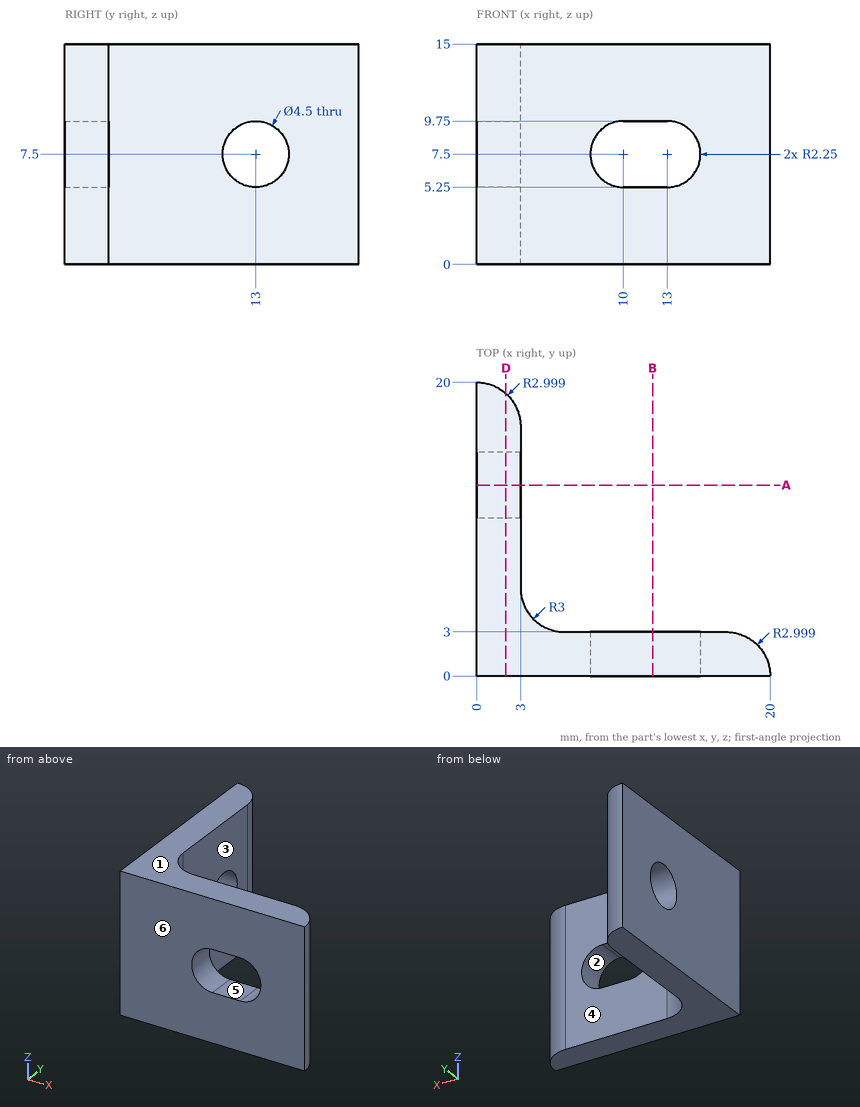
Geometry: see drawing. Coordinates: mm, zero at the bounding-box minimum. A direction names the side the tool comes from. Coordinates: 2 decimals unless noted, no trailing zeros. Loops run counter-clockwise (first coordinate to the right, second up) from the corner with the lowest first, then second, coordinate; pieces in that order, holes last. Notation, with made-up numbers: M -17,17.25 L 14,17.25 A8 ccw 14,29.25 Z; hole C 89.25,3.5 d11. An arc over 180 degrees is marked long. Answer in a Markdown table with one row per item.
Q1. First-contact query: pin 1 (4 mm diameter, centred on y = 15, z = 6, fed in from -X); pin 2 (1 mm diameter, centred on x = 4.5, z = 6, fed in from +Y) (1 decimal). Flat tips, straight axial feed; report the tip coordinate or a pass-through.
Answers below:
| item | result |
|---|---|
| pin 1 | stops at x = 0 |
| pin 2 | stops at y = 3.8 |
Q2. Set-up query: the marked faces 4, 5 and 6. Return all of +Z, -Z, +X, -X, +Y, -Y with unobstructed straight access to the full face (end or side cutting, diameter ignored); none if empty.
Answers below:
| item | result |
|---|---|
| face 4 | +Z, -Z, +X, +Y |
| face 5 | +Y, -Y |
| face 6 | +Z, -Z, +X, -X, -Y |
Q3. Draft query along Z for the marked faces 1, 2 and 3. Return one class per face: pulls with the +Z half, pulls with the -Z half, needs draft (parallel to the pull), parting line crosses it, or undercut.
Answers below:
| item | result |
|---|---|
| face 1 | pulls with the +Z half |
| face 2 | undercut |
| face 3 | needs draft |
Q4. Section A-A on y = 13. Return the cut outline in (x, z), plus the area to 3 significant figures.
Answers below:
| item | result |
|---|---|
| outline | M 0,0 L 3,0 L 3,5.25 L 0,5.25 Z; M 0,9.75 L 3,9.75 L 3,15 L 0,15 Z |
| area | 31.5 mm^2 |
Q5. Ray query, probe 1 along Y at (x, z) = (12.5, 4.25); probe 2 along Y at (x, z) = (0.7, 7.5). Return the intervals inside material, ascending. Write a range as from..to.
Answers below:
| item | result |
|---|---|
| probe 1 | y = 0..3 |
| probe 2 | y = 0..10.75, 15.25..19.92 |
Q6. Section D-D on x = 2. Return the cut outline in (y, z), plus the area to 3 significant figures.
Answers below:
| item | result |
|---|---|
| outline | M 0,0 L 19.24,0 L 19.24,15 L 0,15 Z; hole C 13,7.5 d4.5 |
| area | 273 mm^2 |
